Autodesk Inventor part; units mm, degrees
ref_plane "Work Plane1" through (0, 0, 5) normal (0, 0, 1) x (1, 0, 0)
ref_plane "YZ Plane" through (0, 0, 0) normal (1, 0, 0) x (0, 1, 0)
ref_plane "XZ Plane" through (0, 0, 0) normal (0, 1, 0) x (-1, 0, 0)
sketch "Sketch1" plane through (0, 0, 0) normal (0, 0, 1) x (1, 0, 0)
  line L0 (14.6962, 12.74) -> (14.6962, 0) construction
  line L1 (10.61, 12.2) -> (1.53, 12.2)
  arc A0 (1.53, 12.2) -> (0, 10.67) centre (1.53, 10.67) ccw
  line L2 (0, 10.67) -> (0, 1.53)
  arc A1 (0, 1.53) -> (1.53, 0) centre (1.53, 1.53) ccw
  line L3 (1.53, 0) -> (10.61, 0)
  arc A2 (10.61, 0) -> (12.14, 1.53) centre (10.61, 1.53) ccw
  arc A3 (12.14, 10.67) -> (10.61, 12.2) centre (10.61, 10.67) ccw
  line L4 (12.14, 10.67) -> (12.14, 1.53)
  point P0 (0, 0)
  point P1 (0, 0)
  dimension "d10" = 12.74
ref_plane "Work Plane1" through (0, 0, 5) normal (0, 0, 1) x (1, 0, 0)
sketch "Sketch2" plane through (0, 0, 5) normal (0, 0, 1) x (1, 0, 0)
  line L0 (10.88, 12.74) -> (1.8, 12.74)
  line L1 (10.88, 12.74) -> (1.8, 12.74)
  arc A0 (1.8, 12.74) -> (0, 10.94) centre (1.8, 10.94) ccw
  line L2 (0, 10.94) -> (0, 1.8)
  arc A1 (0, 1.8) -> (1.8, 0) centre (1.8, 1.8) ccw
  line L3 (1.8, 0) -> (10.88, 0)
  arc A2 (10.88, 0) -> (12.68, 1.8) centre (10.88, 1.8) ccw
  line L4 (12.68, 1.8) -> (12.68, 10.94)
  arc A3 (12.68, 10.94) -> (10.88, 12.74) centre (10.88, 10.94) ccw
  circle A4 centre (6.34, 6.37) radius 2.8
  line L5 (5.665, 8.395) -> (7.015, 8.395)
  line L6 (7.015, 4.345) -> (5.665, 4.345)
  line L7 (5.665, 4.345) -> (7.015, 8.395) construction
  line L8 (5.665, 8.395) -> (7.015, 4.345) construction
  line L9 (8.365, 5.695) -> (8.365, 7.045)
  line L10 (4.315, 7.045) -> (4.315, 5.695)
  line L11 (4.315, 5.695) -> (8.365, 7.045) construction
  line L12 (8.365, 5.695) -> (4.315, 7.045) construction
  line L13 (4.315, 5.695) -> (5.665, 5.695)
  line L14 (7.015, 5.695) -> (8.365, 5.695)
  line L15 (5.665, 4.345) -> (5.665, 5.695)
  line L16 (5.665, 7.045) -> (5.665, 8.395)
  line L17 (8.365, 7.045) -> (7.015, 7.045)
  line L18 (5.665, 7.045) -> (4.315, 7.045)
  line L19 (7.015, 8.395) -> (7.015, 7.045)
  line L20 (7.015, 5.695) -> (7.015, 4.345)
  point P0 (0, 0)
  dimension "d3" = 5.6
  dimension "d4" = 4.05
  dimension "d5" = 1.35
  dimension "d6" = 4.05
  dimension "d7" = 1.35
extrude "Extrusion3" add sketch "Sketch1" along normal blind 5
sketch "Sketch3" plane through (0, 0, 5) normal (0, 0, 1) x (1, 0, 0)
  line L0 (10.61, 12.47) -> (1.53, 12.47)
  line L1 (10.61, 12.47) -> (1.53, 12.47)
  arc A0 (1.53, 12.47) -> (-0.27, 10.67) centre (1.53, 10.67) ccw
  line L2 (-0.27, 10.67) -> (-0.27, 1.53)
  arc A1 (-0.27, 1.53) -> (1.53, -0.27) centre (1.53, 1.53) ccw
  line L3 (1.53, -0.27) -> (10.61, -0.27)
  arc A2 (10.61, -0.27) -> (12.41, 1.53) centre (10.61, 1.53) ccw
  line L4 (12.41, 1.53) -> (12.41, 10.67)
  arc A3 (12.41, 10.67) -> (10.61, 12.47) centre (10.61, 10.67) ccw
  circle A4 centre (6.07, 6.1) radius 2.8
  line L5 (5.395, 8.125) -> (6.745, 8.125)
  line L6 (6.745, 4.075) -> (5.395, 4.075)
  line L7 (5.395, 4.075) -> (6.745, 8.125) construction
  line L8 (5.395, 8.125) -> (6.745, 4.075) construction
  line L9 (8.095, 5.425) -> (8.095, 6.775)
  line L10 (4.045, 6.775) -> (4.045, 5.425)
  line L11 (4.045, 5.425) -> (8.095, 6.775) construction
  line L12 (8.095, 5.425) -> (4.045, 6.775) construction
  line L13 (4.045, 5.425) -> (5.395, 5.425)
  line L14 (6.745, 5.425) -> (8.095, 5.425)
  line L15 (5.395, 4.075) -> (5.395, 5.425)
  line L16 (5.395, 6.775) -> (5.395, 8.125)
  line L17 (8.095, 6.775) -> (6.745, 6.775)
  line L18 (5.395, 6.775) -> (4.045, 6.775)
  line L19 (6.745, 8.125) -> (6.745, 6.775)
  line L20 (6.745, 5.425) -> (6.745, 4.075)
  line L21 (10.61, 12.2) -> (1.53, 12.2)
  line L22 (0, 10.67) -> (0, 1.53)
  point P0 (0, 0)
  point P1 (-0.27, -0.27)
  point P2 (6.07, 12.2)
  point P3 (0, 6.1)
  point P4 (6.07, 6.1)
  dimension "d14" = 5.6
  dimension "d15" = 4.05
  dimension "d16" = 1.35
  dimension "d17" = 4.05
  dimension "d18" = 1.35
extrude "Extrusion4" add sketch "Sketch3" along normal blind 4.8 contours A4
sketch "Sketch4" plane through (0, 0, 0) normal (0, 0, -1) x (-1, 0, 0)
  line L0 (-13.9436, 0) -> (-13.9436, 2.266)
  line L1 (-15.5559, 0) -> (-15.5559, 6.84)
  line L2 (-1.53, 0) -> (-10.61, 0)
  line L3 (-7.4059, 5.4445) -> (-4.7341, 5.4445) construction
  line L4 (-4.7341, 5.4445) -> (-4.7341, 2.266) construction
  line L5 (-4.7341, 2.266) -> (-7.4059, 2.266) construction
  line L6 (-7.4059, 2.266) -> (-7.4059, 5.4445) construction
  spline S0 degree 2 poles (-4.9318, 3.2547) (-4.9318, 3.0297) (-5.0974, 2.6615) (-5.2581, 2.5329) knots 0 0 0 1 2 2 2
  spline S1 degree 2 poles (-5.2581, 2.5329) (-5.4187, 2.4044) (-5.8562, 2.266) (-6.1701, 2.266) knots 0 0 0 1 2 2 2
  spline S2 degree 2 poles (-6.1701, 2.266) (-6.526, 2.266) (-7.0352, 2.3846) (-7.1958, 2.4588) knots 0 0 0 1 2 2 2
  line L7 (-7.1958, 2.4588) -> (-7.1958, 3.1212)
  line L8 (-7.1958, 3.1212) -> (-7.1217, 3.1212)
  spline S3 degree 2 poles (-7.1217, 3.1212) (-6.9536, 3.0149) (-6.5013, 2.8567) (-6.3135, 2.8567) knots 0 0 0 1 2 2 2
  spline S4 degree 2 poles (-6.3135, 2.8567) (-6.2022, 2.8567) (-5.9427, 2.8963) (-5.8537, 2.9605) knots 0 0 0 1 2 2 2
  spline S5 degree 2 poles (-5.8537, 2.9605) (-5.7845, 3.0124) (-5.7005, 3.1632) (-5.7005, 3.2991) knots 0 0 0 1 2 2 2
  spline S6 degree 2 poles (-5.7005, 3.2991) (-5.7005, 3.4351) (-5.8191, 3.5809) (-5.918, 3.6155) knots 0 0 0 1 2 2 2
  spline S7 degree 2 poles (-5.918, 3.6155) (-6.0169, 3.6501) (-6.2912, 3.6575) (-6.3975, 3.6575) knots 0 0 0 1 2 2 2
  line L9 (-6.3975, 3.6575) -> (-6.5285, 3.6575)
  line L10 (-6.5285, 3.6575) -> (-6.5285, 4.1939)
  line L11 (-6.5285, 4.1939) -> (-6.4074, 4.1939)
  spline S8 degree 2 poles (-6.4074, 4.1939) (-6.269, 4.1939) (-6.0342, 4.2186) (-5.9526, 4.2557) knots 0 0 0 1 2 2 2
  spline S9 degree 2 poles (-5.9526, 4.2557) (-5.871, 4.2952) (-5.7796, 4.4336) (-5.7796, 4.5523) knots 0 0 0 1 2 2 2
  spline S10 degree 2 poles (-5.7796, 4.5523) (-5.7796, 4.6462) (-5.8661, 4.7624) (-5.9279, 4.7945) knots 0 0 0 1 2 2 2
  spline S11 degree 2 poles (-5.9279, 4.7945) (-6.002, 4.8316) (-6.1998, 4.8563) (-6.269, 4.8563) knots 0 0 0 1 2 2 2
  spline S12 degree 2 poles (-6.269, 4.8563) (-6.3802, 4.8563) (-6.615, 4.8044) (-6.7237, 4.7624) knots 0 0 0 1 2 2 2
  spline S13 degree 2 poles (-6.7237, 4.7624) (-6.8103, 4.7302) (-6.9981, 4.6264) (-7.0426, 4.5992) knots 0 0 0 1 2 2 2
  line L12 (-7.0426, 4.5992) -> (-7.1069, 4.5992)
  line L13 (-7.1069, 4.5992) -> (-7.1069, 5.2517)
  spline S14 degree 2 poles (-7.1069, 5.2517) (-6.9487, 5.3185) (-6.4148, 5.4445) (-6.1355, 5.4445) knots 0 0 0 1 2 2 2
  spline S15 degree 2 poles (-6.1355, 5.4445) (-5.8636, 5.4445) (-5.4632, 5.3506) (-5.3223, 5.2592) knots 0 0 0 1 2 2 2
  spline S16 degree 2 poles (-5.3223, 5.2592) (-5.1666, 5.1628) (-5.0109, 4.8662) (-5.0109, 4.6808) knots 0 0 0 1 2 2 2
  spline S17 degree 2 poles (-5.0109, 4.6808) (-5.0109, 4.4188) (-5.3124, 4.0283) (-5.5596, 3.9714) knots 0 0 0 1 2 2 2
  line L14 (-5.5596, 3.9714) -> (-5.5596, 3.9418)
  spline S18 degree 2 poles (-5.5596, 3.9418) (-5.4509, 3.9269) (-5.2432, 3.8478) (-5.1444, 3.7589) knots 0 0 0 1 2 2 2
  spline S19 degree 2 poles (-5.1444, 3.7589) (-5.0529, 3.6798) (-4.9318, 3.4277) (-4.9318, 3.2547) knots 0 0 0 1 2 2 2
  point P0 (0, 0)
  point P1 (-6.07, 0)
  point P2 (-6.07, 2.266)
  point P3 (-6.07, 6.84)
  point P4 (-6.07, 2.266)
  dimension "d21" = 2.266
  dimension "d22" = 6.84
extrude "Extrusion5" add sketch "Sketch4" along normal blind 0.9
properties part number "IPC 3 key"
Read the model definition and answer for the solid it produces. Units are mm, in the model's axes. A direction names the side the tool comes from. Round coordinates to 2 decimals unless told otherwise and drop trailing zeros. Write each loop counter-clockwise with the first axis right and the second up, starting at its lowest first coordinate (ties: lowest second). Pieces come first, ordered by that corner, then holes.
Q1. The mould has two halves that part along Y. Classify faces 1 (the face through (5, 5.425, 7)), 2 (the face through (0, 6, 2)), 3 (the face through (5.463, 8.833, 7.366)), 4 (the face through (7, 5.425, 7)): released by +Y, released by -Y, zero draft, split by the parting line, or undercut.
Values:
face 1: undercut
face 2: zero draft
face 3: split by the parting line
face 4: undercut
Q2. Find section C-C on x = 1.25. Determine the outline of the cut face in (y, z).
Values:
outline: (0.03, 0) - (12.17, 0) - (12.17, 5) - (0.03, 5) - close
Q3. Find section B-B on y = 6.1. Determine the outline of the cut face in (x, z) (3 decimals).
Values:
outline: (0, 0) - (12.14, 0) - (12.14, 5) - (8.87, 5) - (8.87, 9.8) - (8.095, 9.8) - (8.095, 5) - (4.045, 5) - (4.045, 9.8) - (3.27, 9.8) - (3.27, 5) - (0, 5) - close
Q4. Straight lines are drawn through the part: line 1 (Z direction, x = 2.25, y = 3); line 2 (Z direction, x = 8.75, y = 5.5); line 3 (Y direction, x = 7.75, z = 5.25) (3 decimals). For each, find the intervals that lie inside material, in ascending order.
Values:
line 1: z = 0 to 5
line 2: z = 0 to 9.8
line 3: y = 3.86 to 5.425, 6.775 to 8.34
Q5. Find section D-D on y = 9.75. Determine the outline of the cut face in (x, z), and give its area (3 significant figures).
Values:
outline: (0, 0) - (12.14, 0) - (12.14, 5) - (0, 5) - close
area: 60.7 mm2
Q6. Find section A-A on z = 7.75. Determine the outline of the cut face in (x, y) (3 decimals), and give its area (3 significant figures).
Values:
outline: circle Ø5.6 at (6.07, 6.1); hole (4.045, 5.425) - (5.395, 5.425) - (5.395, 4.075) - (6.745, 4.075) - (6.745, 5.425) - (8.095, 5.425) - (8.095, 6.775) - (6.745, 6.775) - (6.745, 8.125) - (5.395, 8.125) - (5.395, 6.775) - (4.045, 6.775) - close
area: 15.5 mm2
Q7. Flat-ended cylindrical pins translate along their axes: P1, Ø3, axis at y = 8, z = 7, coming from the -X side; P2, Ø0.5, axis at y = 5, z = -0.5, coming from the +X side; P3, Ø1.5, axis at y = 9, z = 3, coming from the -X side; P4, Ø3.5, axis at x = 9, y = 8.5, coming from the -Z side. Find the tip coordinate at first contact, or state that the pin passes through.
Values:
P1: stops at x = 3.3
P2: stops at x = 7.11
P3: stops at x = 0
P4: stops at z = 0
Q8. A tool of negligible diameter and unlimited length cuts with its end or side. For faces 5 (the face through (8.095, 6, 7)), 6 (the face through (0.5, 0.4, 2.5)), from which of +Z, -Z, +X, -X, +Y, -Y can it reach the whole face along a straight path? Write none if from no direction.
Values:
face 5: +Z
face 6: +Z, -Z, -X, -Y
